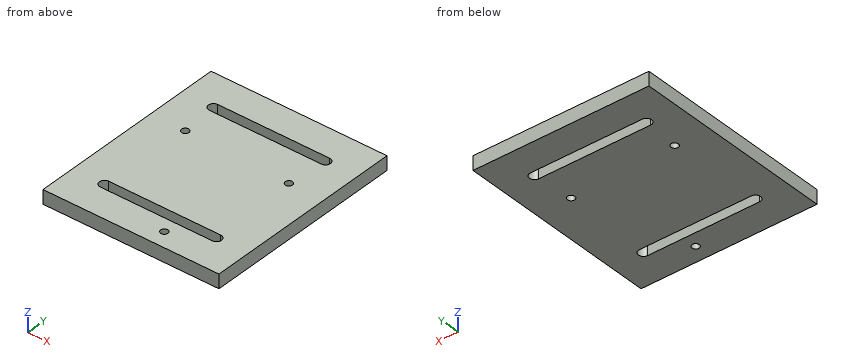
```python
from build123d import *

# Parameters (mm, degrees)
SKETCH1_W           = 80
SKETCH1_H           = 92.5
SKETCH1_R           = 1.65
BOSS_EXTRUDE2_DEPTH = 6.35


with BuildPart() as part:
    # Sketch1 → Boss-Extrude2 (new body)
    with BuildSketch(Plane.XY):
        Rectangle(SKETCH1_W, SKETCH1_H)
        with Locations((-24.08, 12.8)):
            Circle(SKETCH1_R, mode=Mode.SUBTRACT)
        with Locations((24.08, 11.53)):
            Circle(SKETCH1_R, mode=Mode.SUBTRACT)
        with Locations((8.94, -38.71)):
            Circle(SKETCH1_R, mode=Mode.SUBTRACT)
        with BuildLine():
            Line((-25.454545455, 32.285), (25.454545455, 32.285))
            ThreePointArc((25.454545455, 32.285), (27.739545455, 30), (25.454545455, 27.715))
            Line((25.454545455, 27.715), (-25.454545455, 27.715))
            ThreePointArc((-25.454545455, 27.715), (-27.739545455, 30), (-25.454545455, 32.285))
        make_face(mode=Mode.SUBTRACT)
        with BuildLine():
            Line((-25.454545455, -27.715), (25.454545455, -27.715))
            ThreePointArc((25.454545455, -27.715), (27.739545455, -30), (25.454545455, -32.285))
            Line((25.454545455, -32.285), (-25.454545455, -32.285))
            ThreePointArc((-25.454545455, -32.285), (-27.739545455, -30), (-25.454545455, -27.715))
        make_face(mode=Mode.SUBTRACT)
    extrude(amount=BOSS_EXTRUDE2_DEPTH)


solid = part.part
```
Geometry check sheet. Reference: the model listing, model coordinates, mm. Give positions to 0.01 mm unless a question says otherwise; leave off trailing zeros. Loops run counter-clockwise (first coordinate to the right, second up) from the corner with the lowest first, then second, coordinate; pieces in that order, holes last. Notation, with made-up numbers: M 65,-6.75 L 77,-6.75 A20 ccw 77,17.25 Z; hole C -22,18.25 d7. An arc over 180 degrees is marked long. Write item = value, one per line.
(1) Material ranges on line 1 (Y direction, x = 24.08, z = 3.5) (3 decimals); line 2 (Y direction, x = -3, z = 2.25) (3 decimals); line 3 (Y direction, x = -24.08, z = 3) (3 decimals), recorded low to high. Write a range as [from, to].
Answer below:
line_1 = [-46.25, -32.285], [-27.715, 9.88], [13.18, 27.715], [32.285, 46.25]
line_2 = [-46.25, -32.285], [-27.715, 27.715], [32.285, 46.25]
line_3 = [-46.25, -32.285], [-27.715, 11.15], [14.45, 27.715], [32.285, 46.25]
(2) Sectioned sample at B-B, the plane y = -38.71. Record the cut outline in (x, z).
Answer below:
outline = M -40,0 L 7.29,0 L 7.29,6.35 L -40,6.35 Z; M 10.59,0 L 40,0 L 40,6.35 L 10.59,6.35 Z
(3) Sectioned sample at A-A, the plane x = 24.08. Record the cut outline in (y, z) (3 decimals).
Answer below:
outline = M -46.25,0 L -32.285,0 L -32.285,6.35 L -46.25,6.35 Z; M -27.715,0 L 9.88,0 L 9.88,6.35 L -27.715,6.35 Z; M 13.18,0 L 27.715,0 L 27.715,6.35 L 13.18,6.35 Z; M 32.285,0 L 46.25,0 L 46.25,6.35 L 32.285,6.35 Z
(4) Sectioned sample at D-D, the plane x = 2.5. Record the cut outline in (y, z) (3 decimals).
Answer below:
outline = M -46.25,0 L -32.285,0 L -32.285,6.35 L -46.25,6.35 Z; M -27.715,0 L 27.715,0 L 27.715,6.35 L -27.715,6.35 Z; M 32.285,0 L 46.25,0 L 46.25,6.35 L 32.285,6.35 Z
(5) Sectioned sample at C-C, the plane z = 2. Record the cut outline in (x, y) (3 decimals).
Answer below:
outline = M -40,-46.25 L 40,-46.25 L 40,46.25 L -40,46.25 Z; hole C -24.08,12.8 d3.3; hole M -25.455,-32.285 L 25.455,-32.285 A2.285 ccw 25.455,-27.715 L -25.455,-27.715 A2.285 ccw Z; hole M -25.455,27.715 L 25.455,27.715 A2.285 ccw 25.455,32.285 L -25.455,32.285 A2.285 ccw Z; hole C 8.94,-38.71 d3.3; hole C 24.08,11.53 d3.3
